Part print with two shaded views. Sizes in mm from the minimum x, y, z corner. Coordinates: 2 decimals unless noted, no trailing zeros. Write each loop counter-clockwise with the first axis right and the second up, starting at its lowest first coordinate (ties: lowest second). Pieces come first, ordered by that corner, then holes.
Q1. Pin check, flat tips, straight feed: P1, Ø1.5, axis at x = 9, y = 2, coming from the -Z side (1 decimal); P2, Ø3, axis at x = 12.5, z = 24.5, coming from the -Y side; P3, Ø6, axis at x = 10, z = 30.5, coming from the -Y side. Stop position of each tip, or through.
Q2. Band-saw the part on A-A, the plane z = 29.5. Write the cut outline in (x, y) (1 decimal).
Q3. Drill centre lines: probe 1 along Z at (x, y) = (13.5, 2.55) (1 decimal); probe 2 along X at (y, z) = (1.55, 7.5) (1 decimal); probe 3 along X at (y, z) = (2.1, 15.5) (1 decimal). Where is each one in solid material? Low to high.
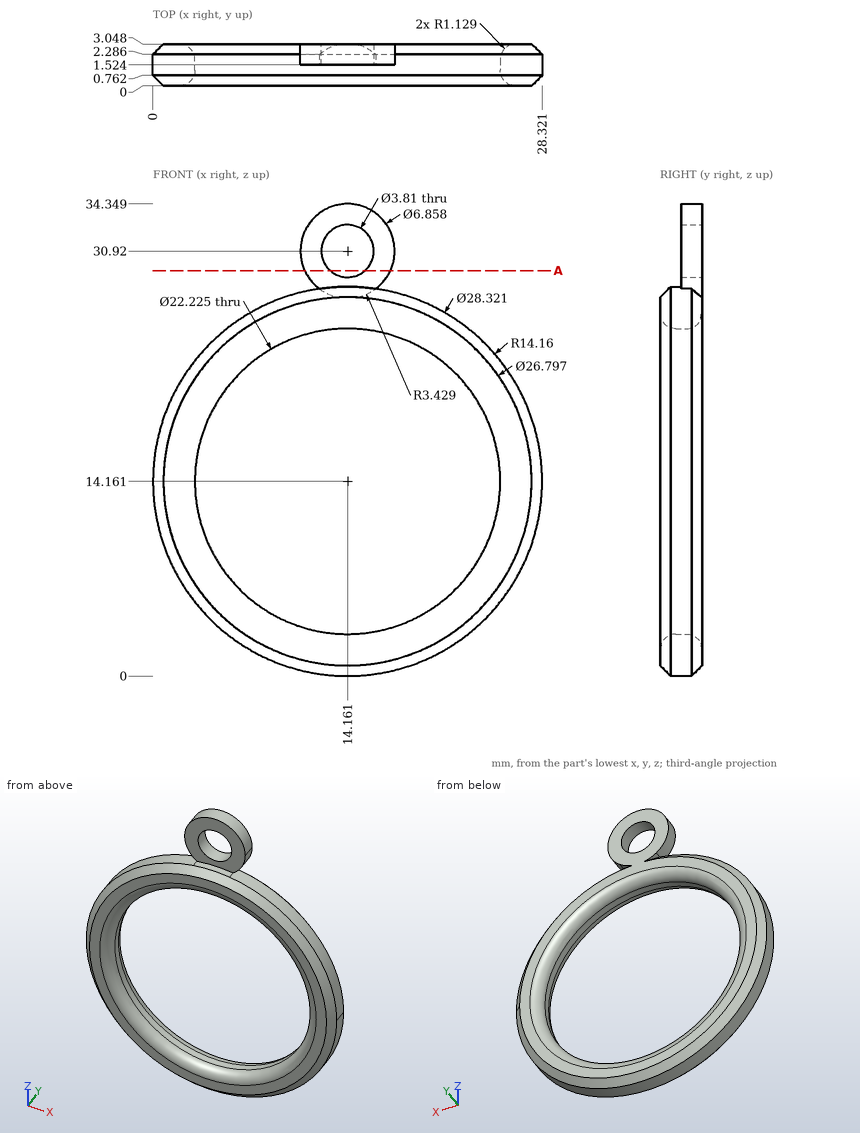
Answer sheet:
1. P1: stops at z = 0.7
1. P2: stops at y = 0.03
1. P3: stops at y = 0.46
2. outline: (11, 1.5) - (12.9, 1.5) - (12.9, 3) - (11, 3) - close; (15.4, 1.5) - (17.3, 1.5) - (17.3, 3) - (15.4, 3) - close
3. probe 1: z = 0.3 to 2.9, 25.4 to 29.1, 32.7 to 34.3
3. probe 2: x = 1.7 to 5.3, 23.1 to 26.7
3. probe 3: x = 0.1 to 3.1, 25.2 to 28.3
